Can you work these out from the model? Positions are in its coordinate system, mm. Give positions to 0.01 mm unless a question says otherwise; leave off trailing zeros. Write each loop counter-clockwise with the first axis right and the second up, starting at its lowest first coordinate (ties: lowest second). Pieces come first, ordered by that corner, then holes. Notation, with made-up numbers: (87, 85.25) - (111, 85.25) arc R22 ccw to (111, 94.25) - close; hole circle Ø8 at (23.5, 66). An arc over 180 degrees is marked (long way). Return JSON: item names as keys, results as strings. Group by question number.
Autodesk Inventor part; units mm, degrees
ref_plane "YZ Plane" through (0, 0, 0) normal (1, 0, 0) x (0, 1, 0)
ref_plane "XZ Plane" through (0, 0, 0) normal (0, 1, 0) x (-1, 0, 0)
ref_plane "XY Plane" through (0, 0, 0) normal (0, 0, 1) x (1, 0, 0)
sketch "Sketch4" plane through (0, 0, 0) normal (0, 0, 1) x (1, 0, 0)
  line L0 (92.7325, 70.7032) -> (-95.1675, 70.7032)
  arc A0 (-95.1675, 70.7032) -> (-99.1675, 66.7032) centre (-95.1675, 66.7032) ccw
  line L1 (-99.1675, 66.7032) -> (-99.1675, -37.2051)
  arc A1 (-91.7887, 67.4724) -> (-95.6675, 64.7032) centre (-94.1675, 66.7032) ccw
  line L2 (-99.1675, -37.2051) -> (-79.7175, -37.2051)
  arc A2 (-77.7175, -39.2051) -> (-79.7175, -37.2051) centre (-79.7175, -39.2051) ccw
  line L3 (-77.7175, -39.2051) -> (-77.7175, -50.6763)
  line L4 (-77.7175, -50.6763) -> (-67.7175, -67.9968)
  line L5 (-67.7175, -67.9968) -> (82.2825, -67.9968)
  circle A3 centre (-71.0649, -52.9681) radius 2.5
  line L6 (82.2825, -67.9968) -> (92.2825, -50.6763)
  circle A4 centre (86.0549, -52.9681) radius 2.5
  line L7 (92.2825, -50.6763) -> (92.2825, -39.2051)
  arc A5 (94.2825, -37.2051) -> (92.2825, -39.2051) centre (94.2825, -39.2051) ccw
  line L8 (94.2825, -37.2051) -> (96.7325, -37.2051)
  line L9 (96.7325, -37.2051) -> (96.7325, 66.7032)
  arc A6 (96.7325, 66.7032) -> (92.7325, 70.7032) centre (92.7325, 66.7032) ccw
  arc A7 (93.3598, 64.019) -> (90.8929, 68.2807) centre (92.5018, 66.3672) ccw
  arc A8 (90.8929, 68.2807) -> (93.3598, 64.019) centre (92.5018, 66.3672) ccw
  arc A9 (-95.6675, 64.7032) -> (-91.7887, 67.4724) centre (-94.1675, 66.7032) ccw
  point P0 (0, 0)
extrude "Extrusion4" add sketch "Sketch4" along normal blind 2
fillet "Fillet1" radius 5 6 edges at (-99.1675, -37.2051, 1) (-77.7175, -50.6763, 1) (-67.7175, -67.9968, 1) (82.2825, -67.9968, 1) (92.2825, -50.6763, 1) (96.7325, -37.2051, 1)
sketch "Sketch5" plane through (0, 0, 2) normal (0, 0, 1) x (1, 0, 0)
  circle A0 centre (-46.9967, 41.5331) radius 20
  circle A1 centre (-46.9967, 41.5331) radius 11
  point P0 (0, 0)
  dimension "d12" = 40
  dimension "d13" = 22
extrude "Extrusion5" cut sketch "Sketch5" against normal blind 10
sketch "Sketch6" plane through (0, 0, 2) normal (0, 0, 1) x (1, 0, 0)
  arc A0 (-46.4486, 64.74) -> (-47.34, 46.911) centre (-41.9812, 55.5798) ccw
  arc A1 (-38.695, 63.3) -> (-44.2546, 45.6452) centre (-40.3973, 54.1333) ccw
  line L0 (-47.34, 46.911) -> (-44.2546, 45.6452)
  line L1 (-46.4486, 64.74) -> (-38.695, 63.3)
  point P0 (0, 0)
extrude "Extrusion6" add sketch "Sketch6" against normal up to surface (2 mm away)
pattern_circular "Circular Pattern1" count 6 over 360 about axis through (-46.9967, 41.5331, 2) along (0, 0, -1) of "Extrusion6"
sketch "Sketch7" plane through (0, 0, 2) normal (0, 0, 1) x (1, 0, 0)
  line L0 (-95.1675, 71.7032) -> (92.7325, 71.7032)
  line L1 (92.7325, 70.7032) -> (-95.1675, 70.7032)
  arc A0 (-95.1675, 70.7032) -> (-99.1675, 66.7032) centre (-95.1675, 66.7032) ccw
  arc A1 (-95.1675, 71.7032) -> (-99.1675, 66.7032) centre (-94.4287, 67.0121) ccw
  arc A2 (96.7325, 66.7032) -> (92.7325, 70.7032) centre (92.7325, 66.7032) ccw
  arc A3 (96.7325, 66.7032) -> (92.7325, 71.7032) centre (91.9937, 67.0121) ccw
  point P0 (0, 0)
extrude "Extrusion7" add sketch "Sketch7" against normal up to surface (2 mm away)
properties part number "Back Plate"
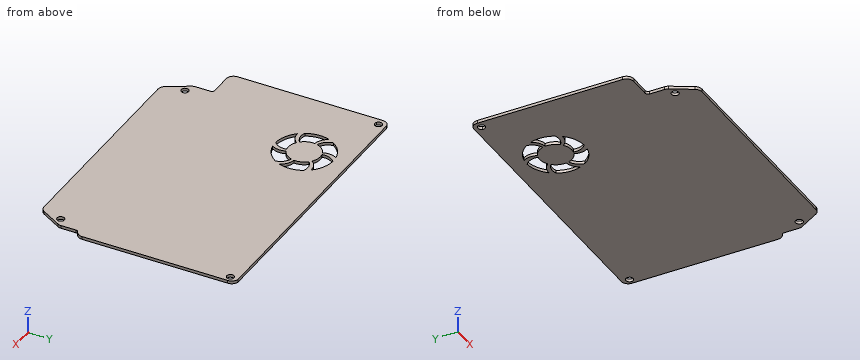
1) Imagine slicing it at B-B, the plane z = 0.4. Count the separate pieces of the cut face and the enclosed holes in it, and give its area (3 significant figures).
2) Imagine slicing it at A-A, the plane x = -86. Write out the boundary of the cut face in (y, z).
3) I need wall thicknesses on line 1 along X through (y, z) = (33, 1.1); line 2 along X through (y, z) = (16, 0.25); line 3 along X through (y, z) = (39, 0.55). Which ranges of each line are inside material? Lowest first, please.
4) Will these pins go through, and if not, where does the flat tip stop? pin 1 Ø4.5 at (x, y) = (92.5, 66.37) entering from -Z; pin 2 Ø0.6 at (y, z) = (-42.5, 0.5) entering from -X; pin 3 Ø1 at (x, z) = (-86, 1.5) entering from -Y.
Resolved:
{
 "1": {"separate pieces": "1", "enclosed holes": "10", "area": "25,600 mm^2"},
 "2": {"outline": "(-37.21, 0) - (71.7, 0) - (71.7, 2) - (-37.21, 2) - close"},
 "3": {"line 1": "-99.17 to -65.08, -56.33 to -40.06, -30.74 to 96.73", "line 2": "-99.17 to 96.73", "line 3": "-99.17 to -66.84, -57.7 to -32.26, -27.16 to 96.73"},
 "4": {"pin 1": "through", "pin 2": "x = -77.72", "pin 3": "y = -37.21"}
}
